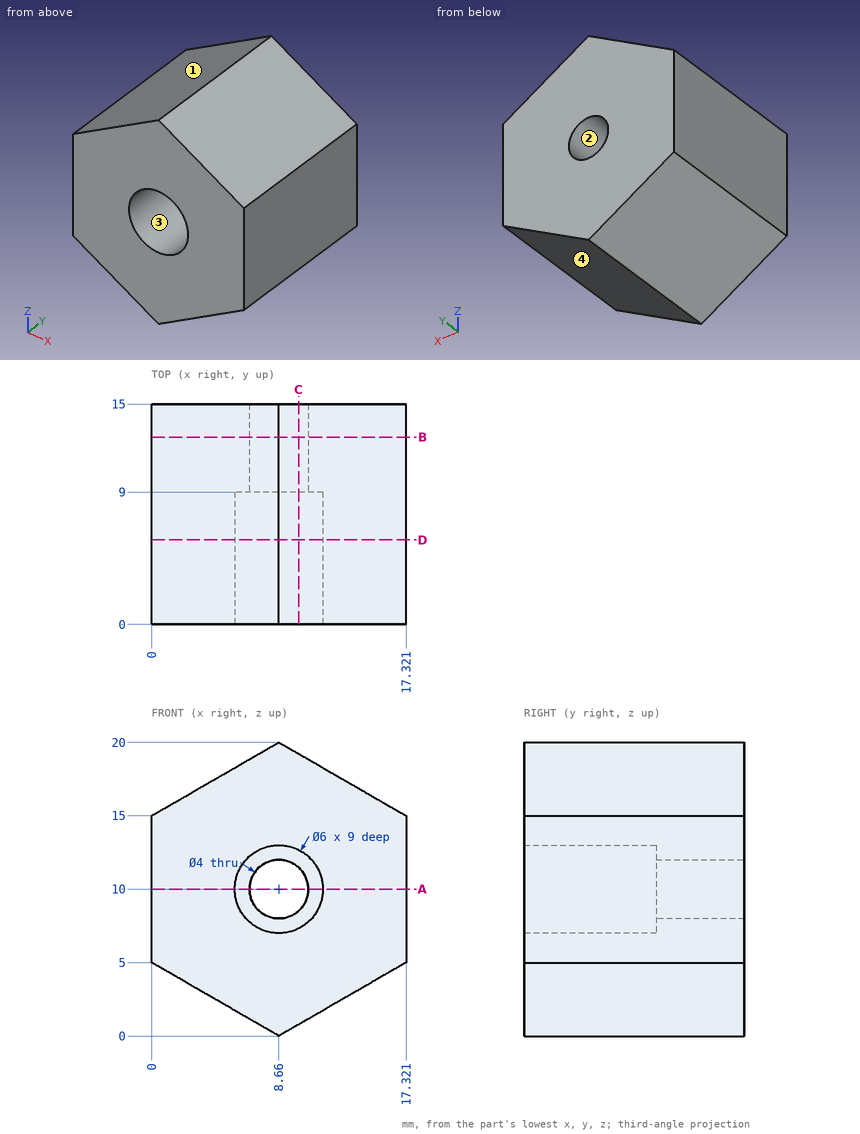
Answer from the drawing. Dimensions are ordinates in mm from the lowest x, y and z of the part. Coordinates: 2 decimals unless noted, no trailing zeros. Loops run counter-clockwise (first coordinate to the right, second up) from the corner with the lowest first, then second, coordinate; pieces in that order, holes last. Notation, with made-up numbers: (55.25, 8.5) - (114.25, 8.5) arc R9 cw to (114.25, 17.5) - close; hole circle Ø8 at (-0.5, 65.25). An arc over 180 degrees is marked (long way). Use a Markdown table: item, result.
Item 1: Find section D-D, the plane y = 5.75. Determine the outline of the cut face in (x, z).
Evaluation:
| item | result |
|---|---|
| outline | (0, 5) - (8.66, 0) - (17.32, 5) - (17.32, 15) - (8.66, 20) - (0, 15) - close; hole circle Ø6 at (8.66, 10) |
Item 2: Find section B-B, the plane y = 12.75. Determine the outline of the cut face in (x, z).
Evaluation:
| item | result |
|---|---|
| outline | (0, 5) - (8.66, 0) - (17.32, 5) - (17.32, 15) - (8.66, 20) - (0, 15) - close; hole circle Ø4 at (8.66, 10) |
Item 3: Consider probe 1 along X at (y, z) = (5.25, 10); probe 2 along X at (y, z) = (10.3, 10); probe 3 along Z at (x, y) = (9.75, 13.25) (1 decimal). Determine where each line is inside the solid, lowest interval first. Write a range as from..to.
Evaluation:
| item | result |
|---|---|
| probe 1 | x = 0..5.66, 11.66..17.32 |
| probe 2 | x = 0..6.66, 10.66..17.32 |
| probe 3 | z = 0.6..8.3, 11.7..19.4 |
Item 4: Find section C-C, the plane x = 10. Determine the outline of the cut face in (y, z) (1 decimal), and give its area (3 significant figures).
Evaluation:
| item | result |
|---|---|
| outline | (0, 0.8) - (15, 0.8) - (15, 8.5) - (9, 8.5) - (9, 7.3) - (0, 7.3) - close; (0, 12.7) - (9, 12.7) - (9, 11.5) - (15, 11.5) - (15, 19.2) - (0, 19.2) - close |
| area | 211 mm2 |
Item 5: Given pin 1 Ø3 at (x, z) = (10, 9.5) entering from -Y; pin 2 Ø5 at (x, y) = (8.5, 10.5) entering from +Z; pin 3 Ø6 at (x, y) = (2.5, 6.5) entering from -Z (1 decimal); pin 4 Ø3 at (x, z) = (8.66, 10) entering from -Y, each flat-ended and moving along its own axis, determine where each tip first touches the part or whether it passes through.
Evaluation:
| item | result |
|---|---|
| pin 1 | stops at y = 9 |
| pin 2 | stops at z = 20 |
| pin 3 | stops at z = 1.8 |
| pin 4 | passes through |
Item 6: Find section A-A, the plane z = 10. Determine the outline of the cut face in (x, y).
Evaluation:
| item | result |
|---|---|
| outline | (0, 0) - (5.66, 0) - (5.66, 9) - (6.66, 9) - (6.66, 15) - (0, 15) - close; (10.66, 9) - (11.66, 9) - (11.66, 0) - (17.32, 0) - (17.32, 15) - (10.66, 15) - close |
Item 7: The mould has two halves that part along X. Classify the marked faces 1, 2, 3 and 4: +X half, -X half, draft (parallel to the pull), parting line (faces both ways), or undercut.
Evaluation:
| item | result |
|---|---|
| face 1 | -X half |
| face 2 | undercut |
| face 3 | undercut |
| face 4 | +X half |
